Can you work these out from the drawing? Everything is in mm from the part's minimum corner. A direction names the side the tool comes from. Give positions to 0.01 mm unless a question says otherwise; leave off trailing zeros. Write each loop counter-clockwise with the first axis right and the second up, starting at its lowest first coordinate (ties: lowest second). Pieces come first, ordered by that corner, then holes. Notation, with made-up numbers: (8, 0) - (51, 0) arc R29 ccw to (51, 35) - close; hole circle Ø1 at (-33, 72.5). An arc over 180 degrees is marked (long way). Answer in a Markdown table with one row per item.
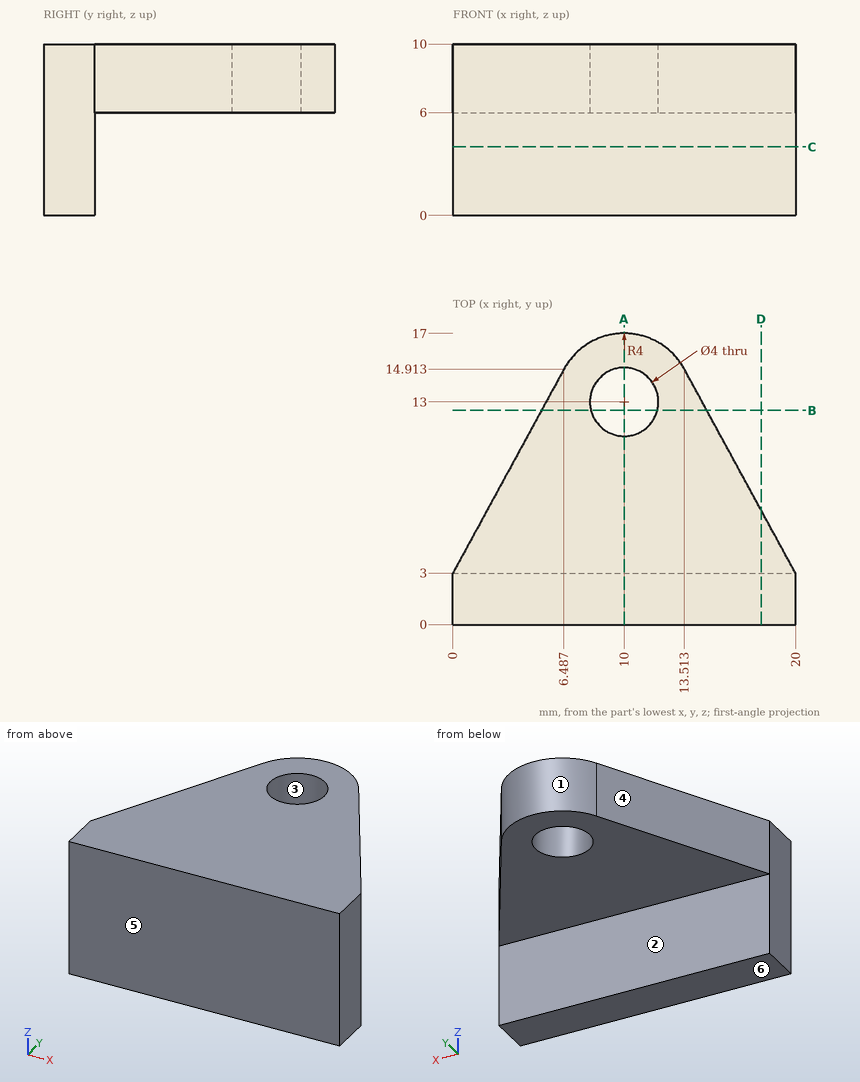
1) If I drill on line 1 (Y direction, x = 16.5, z = 5.75); line 2 (Z direction, x = 6.75, y = 14.5); line 3 (X direction, y = 12.25, z = 9.25), over which ranges is the centre line in solid material (lowest first)?
Check values:
| item | result |
|---|---|
| line 1 | y = 0 to 3 |
| line 2 | z = 6 to 10 |
| line 3 | x = 5.04 to 8.15, 11.85 to 14.96 |
2) Imagine slicing it at A-A (x = 10). List the corners of the cut face in (y, z) for me, then the cut area to 3 significant figures.
Check values:
| item | result |
|---|---|
| outline | (0, 0) - (3, 0) - (3, 6) - (11, 6) - (11, 10) - (0, 10) - close; (15, 6) - (17, 6) - (17, 10) - (15, 10) - close |
| area | 70.0 mm2 |
3) On a 3-axis mill with a long thin cutter (end or side, diameter ignored), from which of +Z, -Z, +X, -X, +Y, -Y can I reach the whole of each face in a straight line? I mean the marked faces 1 and 2. Say none if no direction works.
Check values:
| item | result |
|---|---|
| face 1 | +Z, -Z, +Y |
| face 2 | -Z, +X, -X, +Y |
4) Imagine slicing it at C-C (z = 4). List the corners of the cut face in (x, y) for me.
Check values:
| item | result |
|---|---|
| outline | (0, 0) - (20, 0) - (20, 3) - (0, 3) - close |
5) Imagine slicing it at D-D (x = 18). List the corners of the cut face in (y, z) for me, then the cut area to 3 significant figures.
Check values:
| item | result |
|---|---|
| outline | (0, 0) - (3, 0) - (3, 6) - (6.67, 6) - (6.67, 10) - (0, 10) - close |
| area | 44.7 mm2 |
6) Imagine slicing it at B-B (y = 12.5). List the corners of the cut face in (x, z) for me.
Check values:
| item | result |
|---|---|
| outline | (5.17, 6) - (8.06, 6) - (8.06, 10) - (5.17, 10) - close; (11.94, 6) - (14.83, 6) - (14.83, 10) - (11.94, 10) - close |
7) We'd pull the mould along Y, two halves only. Please class the marked faces 3, 4, 5 and 6: +Y half, -Y half, draft (parallel to the pull), parting line (faces both ways), or undercut.
Check values:
| item | result |
|---|---|
| face 3 | undercut |
| face 4 | +Y half |
| face 5 | -Y half |
| face 6 | draft |
8) Will these pins go through, and if not, where does the flat tip stop? P1, Ø4, axis at x = 17.5, z = 8.5, coming from the -Y side; P2, Ø6, axis at x = 2.5, y = 10.5, coming from the -Z side; P3, Ø1.8, axis at x = 13.5, z = 3, coming from the +Y side.
Check values:
| item | result |
|---|---|
| P1 | stops at y = 0 |
| P2 | stops at z = 6 |
| P3 | stops at y = 3 |
